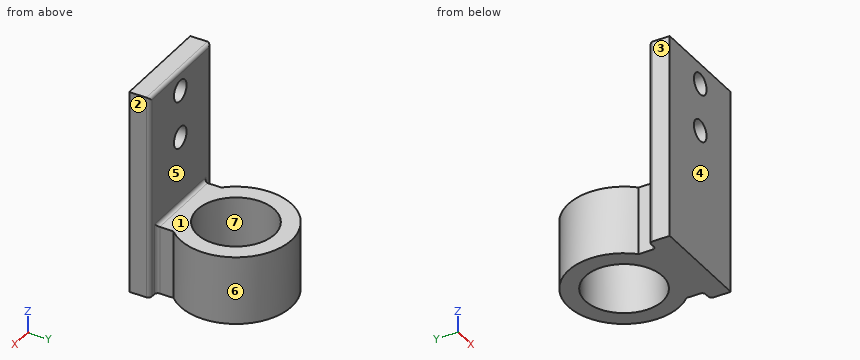
Autodesk Fusion 360 part; units mm, degrees
sketch "Sketch1" plane through (0, 0, 0) normal (0, 0, 1) x (1, 0, 0)
  line L0 (0, 0) -> (15, 0)
  line L1 (15, 0) -> (15, 3)
  line L2 (15, 3) -> (0, 3)
  line L3 (0, 3) -> (0, 0)
  line L4 (1.6263, 3) -> (13.3737, 3)
  line L5 (13.3737, 3) -> (13.3737, 5.5)
  line L6 (13.3737, 5.5) -> (1.6263, 5.5)
  line L7 (1.6263, 5.5) -> (1.6263, 3)
  circle A0 centre (7.5, 11.15) radius 8.15
  circle A1 centre (7.5, 11.15) radius 5.65
  line L8 (7.5, 0) -> (7.5, 3) construction
  line L9 (7.5, 5.5) -> (7.5, 3) construction
  dimension "d1" = 11.3
  dimension "d2" = 15
  dimension "d4" = 3
  dimension "d19" = 2.5
extrude "Extrude1" add sketch "Sketch1" along normal blind 10 contours L2 L4 L7 A0 | L2 L4 L5 A0 | L6 A0 | L6 A0
extrude "Extrude2" add sketch "Sketch1" along normal blind 30 contours L0 L1 L2 L3 L4
sketch "Sketch2" plane through (0, 3, 0) normal (0, 1, 0) x (-1, 0, 0)
  line L0 (-13.3737, 0) -> (-13.3737, 10)
  line L1 (-13.3737, 10) -> (-1.6263, 10)
  line L2 (-1.6263, 10) -> (-1.6263, 0)
  line L3 (-1.6263, 0) -> (0, 0)
  line L4 (0, 0) -> (0, 30)
  line L5 (0, 30) -> (-15, 30)
  line L6 (-15, 30) -> (-15, 0)
  line L7 (-15, 0) -> (-13.3737, 0)
  line L8 (-7.5, 30) -> (-7.5, 10) construction
  circle A0 centre (-7.5, 27) radius 1.55
  circle A1 centre (-7.5, 20) radius 1.55
  dimension "d9" = 3.1
  dimension "d10" = 3.1
  dimension "d11" = 7
  dimension "d12" = 3
extrude "Extrude3" cut sketch "Sketch2" against normal up to surface (3 mm away) contours A0 | A1
fillet "Fillet1" radius 0.5 3 edges at (0, 3, 15) (7.5, 3, 30) (15, 3, 15)
fillet "Fillet2" radius 0.5 3 edges at (13.3737, 3, 5) (7.5, 3, 10) (1.6263, 3, 5)
equation "d10 = d9"
Source: CAD feature listing. Evaluate the final solid. Frame: model axes, mm. Face numbers are marked on the shaded views. A direction names the side the tool comes from. Coordinates: 2 decimals unless noted, no trailing zeros. Order: outer loops, then holes, each group sorted by start corner. A loop starts at its lowest first (then second) coordinate and runs counter-clockwise, first axis right, second up. Notation, with made-up numbers: M 57,29 L 95,29 A26 cw 95,68 Z; hole C 4,-21.75 d11. An arc over 180 degrees is marked long. Write each question's results on one line, items separated by ' | '. Start each with the question number.
Item 1: Cut plane B-B (y = 11.15). Return loops of the section in (x, z).
Item 2: Cut plane D-D (y = 2). Return loops of the section in (x, z).
Item 3: Set-up query: the marked faces 1, 2, 3 and 4. Return all of +Z, -Z, +X, -X, +Y, -Y with unobstructed straight access to the full face (end or side cutting, diameter ignored); none if empty.
Item 4: Line query: probe 1 along Z at (x, y) = (7.5, 1.35); probe 2 along Y at (x, z) = (7.5, 3); probe 3 along Y at (x, z) = (6, 16). Output: solid intervals per line, ascending.
Item 5: Cut plane A-A (x = 7.5). Return loops of the section in (y, z).
Item 6: Draft query along X for the marked faces 5, 6 and 7. Return one class per face: pulls with the +X half, pulls with the -X half, needs draft (parallel to the pull), parting line crosses it, or undercut.
Item 7: First-contact query: pin 1 Ø2 at (x, y) = (1, 8) entering from +Z; pin 2 Ø3 at (y, z) = (1, 8.5) entering from -X; pin 3 Ø3 at (y, z) = (0.5, 12) entering from +X. Flat tips, straight axial feed; report the tip coordinate or a pass-through.
Item 8: Cut plane C-C (z = 27). Return loops of the section in (x, y).
Checked values:
1) outline: M -0.65,0 L 1.85,0 L 1.85,10 L -0.65,10 Z; M 13.15,0 L 15.65,0 L 15.65,10 L 13.15,10 Z
2) outline: M 0,0 L 15,0 L 15,30 L 0,30 Z; hole C 7.5,20 d3.1; hole C 7.5,27 d3.1
3) face 1: +Z, +X, -X, +Y | face 2: +Z, -Z, +X, -Y | face 3: +Z, -Z, -X, -Y | face 4: +Z, -Z, +X, -X, -Y
4) probe 1: z = 0 to 18.45, 21.55 to 25.45, 28.55 to 30 | probe 2: y = 0 to 5.5, 16.8 to 19.3 | probe 3: y = 0 to 3
5) outline: M 0,0 L 5.5,0 L 5.5,10 L 3.5,10 A0.5 cw 3,10.5 L 3,18.45 L 0,18.45 Z; M 0,21.55 L 3,21.55 L 3,25.45 L 0,25.45 Z; M 0,28.55 L 3,28.55 L 3,29.5 A0.5 ccw 2.5,30 L 0,30 Z; M 16.8,0 L 19.3,0 L 19.3,10 L 16.8,10 Z
6) face 5: needs draft | face 6: parting line crosses it | face 7: undercut
7) pin 1: stops at z = 10 | pin 2: stops at x = 0 | pin 3: stops at x = 15
8) outline: M 0,0 L 5.95,0 L 5.95,3 L 0.5,3 A0.5 ccw 0,2.5 Z; M 9.05,0 L 15,0 L 15,2.5 A0.5 ccw 14.5,3 L 9.05,3 Z
